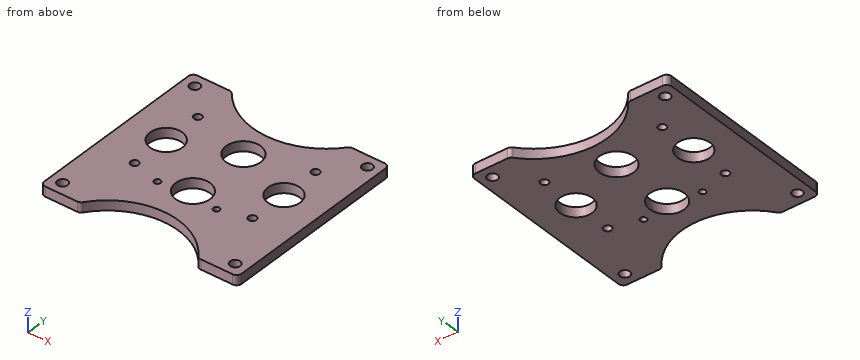
Autodesk Inventor part; units mm, degrees
ref_plane "YZ Plane" through (0, 0, 0) normal (1, 0, 0) x (0, 1, 0)
ref_plane "XZ Plane" through (0, 0, 0) normal (0, 1, 0) x (-1, 0, 0)
ref_plane "XY Plane" through (0, 0, 0) normal (0, 0, 1) x (1, 0, 0)
ref_plane "Work Plane1" through (-63.5, 101.6, 34.925) normal (0, 0, 1) x (1, 0, 0)
sketch "Sketch2" plane through (-63.5, 101.6, 34.925) normal (0, 0, 1) x (1, 0, 0)
  circle A0 centre (63.5, -101.6) radius 11.1125
  circle A1 centre (44.45, -106.3625) radius 2.0193
  circle A2 centre (44.45, -106.3625) radius 2.0193
  circle A3 centre (25.5848, -101.08) radius 2.54
  circle A4 centre (25.5848, -101.08) radius 2.54
  line L0 (44.45, -106.3625) -> (82.55, -106.3625)
  circle A5 centre (82.55, -106.3625) radius 2.0193
  circle A6 centre (101.4152, -101.08) radius 2.54
  line L1 (25.5848, -101.08) -> (101.4152, -101.08)
  circle A7 centre (101.4152, -101.08) radius 2.54
  line L2 (25.5848, -101.08) -> (25.5848, -75.68)
  line L3 (101.4152, -101.08) -> (101.4152, -75.68)
  circle A8 centre (25.5848, -75.68) radius 10.414
  circle A9 centre (101.4152, -75.68) radius 10.414
  circle A10 centre (63.5, -60.9092) radius 11.1125
  line L4 (63.5, -60.9092) -> (63.5, -101.6)
  circle A11 centre (63.5, -60.9092) radius 11.1125
  circle A12 centre (25.5848, -50.28) radius 2.54
  line L5 (25.5848, -50.28) -> (25.5848, -75.68)
  line L6 (101.4152, -75.68) -> (101.4152, -50.28)
  circle A13 centre (25.5848, -50.28) radius 2.54
  circle A14 centre (101.4152, -50.28) radius 2.54
  circle A15 centre (63.5, -101.6) radius 11.1125
  line L7 (127, 0) -> (127, -139.7)
  line L8 (0, -139.7) -> (0, 0)
  line L9 (0, -144.9324) -> (127, -144.9324)
  line L10 (0, -144.9324) -> (7.9248, -144.9324)
  line L11 (7.9248, -144.9324) -> (7.9248, -137.0076)
  circle A16 centre (7.9248, -137.0076) radius 3.2512
  line L12 (127, -144.9324) -> (119.0752, -144.9324)
  line L13 (119.0752, -144.9324) -> (119.0752, -137.0076)
  circle A17 centre (119.0752, -137.0076) radius 3.2512
  line L14 (0, 0) -> (127, 0)
  line L15 (0, -22.6568) -> (127, -22.6568)
  line L16 (0, -22.6568) -> (7.9248, -22.6568)
  line L17 (7.9248, -22.6568) -> (7.9248, -30.5816)
  line L18 (127, -22.6568) -> (119.0752, -22.6568)
  line L19 (119.0752, -22.6568) -> (119.0752, -30.5816)
  circle A18 centre (7.9248, -30.5816) radius 3.2512
  circle A19 centre (119.0752, -30.5816) radius 3.2512
  line L20 (63.5, 0) -> (63.5, -17.78)
  line L21 (0, -144.9324) -> (0, -22.6568)
  line L22 (127, -144.9324) -> (127, -22.6568)
  line L23 (63.5, -101.6) -> (63.5, -106.3625)
  line L24 (63.5, -106.3625) -> (82.55, -106.3625)
  line L25 (82.55, -106.3625) -> (44.45, -106.3625)
  dimension "d0" = 38.1
  dimension "d1" = 25.4
  dimension "d23" = 7.9248
  dimension "d24" = 7.9248
  dimension "d25" = 17.78
  dimension "d27" = 38.2524
  dimension "d29" = 7.9248
  dimension "d30" = 7.9248
  dimension "d31" = 43.3324
extrude "Extrusion1" add sketch "Sketch2" along normal blind 6.35 contours L7 L22 L9 L21 L8 L15
fillet "Fillet1" radius 3.175 4 edges at (-63.5, 78.9432, 38.1) (-63.5, -43.3324, 38.1) (63.5, 78.9432, 38.1) (63.5, -43.3324, 38.1)
sketch "Sketch5" plane through (-63.5, 101.6, 41.275) normal (0, 0, 1) x (1, 0, 0)
  line L0 (3.175, -144.9324) -> (123.825, -144.9324)
  line L1 (63.5, -144.9324) -> (25.4, -144.9324)
  line L2 (25.4, -144.9324) -> (101.6, -144.9324)
  line L3 (63.5, -144.9324) -> (63.5, -124.6124)
  arc A0 (101.6, -144.9324) -> (25.4, -144.9324) centre (63.5, -170.4912) ccw
  line L4 (123.825, -22.6568) -> (3.175, -22.6568)
  line L5 (25.4, -22.6568) -> (101.6, -22.6568)
  line L6 (63.5, -22.6568) -> (63.5, -41.7068)
  arc A1 (25.4, -22.6568) -> (101.6, -22.6568) centre (63.5, 5.9182) ccw
  line L7 (25.4, -144.9324) -> (101.6, -144.9324)
  arc A2 (101.6, -144.9324) -> (25.4, -144.9324) centre (63.5, -170.4912) ccw
  point P0 (63.5, -101.6)
  dimension "d16" = 38.1
  dimension "d17" = 76.2
  dimension "d18" = 20.32
  dimension "d19" = 19.05
extrude "Extrusion2" cut sketch "Sketch5" against normal blind 25.4
fillet "Fillet2" radius 3.175 4 edges at (-38.1, 78.9432, 38.1) (38.1, 78.9432, 38.1) (38.1, -43.3324, 38.1) (-38.1, -43.3324, 38.1)
properties part number "am-2725+3CIM4U+Motor+Plate+r2" material "Aluminum 6061"
Work out the finished part from the listing and answer in its coordinate system (mm). Coordinates: 2 decimals unless noted, no trailing zeros. Write each loop counter-clockwise with the first axis right and the second up, starting at its lowest first coordinate (ties: lowest second). Pieces come first, ordered by that corner, then holes.
1. The part is cut by section A-A, the plane x = 0. Write down the section's boundary in (y, z) (1 decimal), and give its area (3 significant figures).
Results list:
outline: (-23, 34.9) - (-11.1, 34.9) - (-11.1, 41.3) - (-23, 41.3) - close; (11.1, 34.9) - (29.6, 34.9) - (29.6, 41.3) - (11.1, 41.3) - close; (51.8, 34.9) - (59.9, 34.9) - (59.9, 41.3) - (51.8, 41.3) - close
area: 244 mm2
2. The part is cut by section B-B, the plane y = 25.92. Write down the section's boundary in (x, z) (3 decimals), and give its area (3 significant figures).
Results list:
outline: (-63.5, 34.925) - (-48.329, 34.925) - (-48.329, 41.275) - (-63.5, 41.275) - close; (-27.501, 34.925) - (27.501, 34.925) - (27.501, 41.275) - (-27.501, 41.275) - close; (48.329, 34.925) - (63.5, 34.925) - (63.5, 41.275) - (48.329, 41.275) - close
area: 542 mm2
3. The part is cut by section D-D, the plane y = -29. Write down the section's boundary in (x, z) (3 decimals), and give its area (3 significant figures).
Results list:
outline: (-63.5, 34.925) - (-22.662, 34.925) - (-22.662, 41.275) - (-63.5, 41.275) - close; (22.662, 34.925) - (63.5, 34.925) - (63.5, 41.275) - (22.662, 41.275) - close
area: 519 mm2
4. The part is cut by section C-C, the plane x = -19.05. Write down the section's boundary in (y, z) (3 decimals), and give its area (3 significant figures).
Results list:
outline: (-27.154, 34.925) - (-6.782, 34.925) - (-6.782, 41.275) - (-27.154, 41.275) - close; (-2.743, 34.925) - (63.869, 34.925) - (63.869, 41.275) - (-2.743, 41.275) - close
area: 552 mm2
5. Consider line 1 along Y through (x, z) = (0, 36.75); line 2 along Y through (x, z) = (-56, 37.25); line 3 along X through (y, z) = (73, 39.25). Determine where each line is inside the solid, lowest interval first.
Results list:
line 1: y = -23.01 to -11.11, 11.11 to 29.58, 51.8 to 59.89
line 2: y = -43.33 to -38.63, -32.18 to 67.8, 74.24 to 78.94
line 3: x = -63.5 to -58.15, -53 to -32.81, 32.81 to 53, 58.15 to 63.5
6. Flat-ended cylindrical pins translate along their axes: pin 1 (6 mm diameter, centred on x = 55.58, y = -35.41, fed in from +Z); pin 2 (1.5 mm diameter, centred on x = -26, z = 36.5, fed in from -Y). Find the tip coordinate at first contact, or state that the pin passes through.
Results list:
pin 1: passes through
pin 2: stops at y = -31.62
